Part model, mm, in its own coordinate system. Give positions to 0.01 mm unless a question says otherwise; leave off trailing zeros. Write each loop counter-clockwise with the first axis right and the second up, starting at its lowest first coordinate (ties: lowest second). Pieces come first, ordered by that corner, then holes.
```python
from build123d import *

# Parameters (mm, degrees)
CROQUIS2_W              = 100
CROQUIS2_H              = 300
SALIENTE_EXTRUIR2_DEPTH = 50


with BuildPart() as part:
    # Croquis2 → Saliente-Extruir2 (new body, symmetric)
    with BuildSketch(Plane.XY):
        Polygon((0, 236.602540378), (50, 150), (-50, 150), align=None)
        Rectangle(CROQUIS2_W, CROQUIS2_H)
        with BuildLine():
            Line((50, -150), (-50, -150))
            ThreePointArc((-50, -150), (0, -200), (50, -150))
        make_face()
    extrude(amount=SALIENTE_EXTRUIR2_DEPTH, both=True)


solid = part.part
```
1) Wall check: L1, parallel to Y at x = -42, z = -5; L2, parallel to Y at x = -41.5, z = -23.5; L3, parallel to X at y = 201, z = 0. Give the ranges that are in metal, low to high.
Answers follow:
L1: y = -177.13 to 163.86
L2: y = -177.89 to 164.72
L3: x = -20.56 to 20.56
2) Saw through at B-B, the plane x = -25.5. Write the cut outline in (y, z).
Answers follow:
outline: (-193.01, -50) - (192.44, -50) - (192.44, 50) - (-193.01, 50) - close
3) Saw through at A-A, the plane z = 34. Write the cut outline in (x, y), then the cut area to 3 significant figures.
Answers follow:
outline: (-50, -150) arc R50 ccw to (50, -150) - (50, 150) - (0, 236.6) - (-50, 150) - close
area: 38,300 mm2
4) Pin check, flat tips, straight feed: pin 1 Ø1 at (x, z) = (-12.5, 25) entering from -Y; pin 2 Ø5 at (x, z) = (1.5, -31) entering from +Y; pin 3 Ø6 at (x, z) = (36, -38.5) entering from +Y. Stop position of each tip, or through.
Answers follow:
pin 1: stops at y = -198.54
pin 2: stops at y = 236.6
pin 3: stops at y = 179.44
5) Saw through at C-C, the plane y = 170.5. Write the cut outline in (x, z).
Answers follow:
outline: (-38.16, -50) - (38.16, -50) - (38.16, 50) - (-38.16, 50) - close
